The model under review builds one solid part; all positions refer to its coordinate system, in mm. A direction names the side the tool comes from. Round coordinates to 2 decimals unless told otherwise and drop trailing zeros. Order: outer loops, then holes, each group sorted by start corner. A loop starts at its lowest first (then second) coordinate and runs counter-clockwise, first axis right, second up.
1) Clearance check with flat-ended pins moving along their axes: P1, Ø10, axis at x = 55, z = -89.5, coming from the +Y side; P2, Ø0.9, axis at x = -4, y = 0, coming from the +Z side; P3, Ø4.5, axis at y = 14, z = -78.5, coming from the +X side. State where each tip first meets the part, or that it passes through.
2) Consider section A-A (y = 20.75). Give the number of separate pieces and of enclosed holes in the cut face, then the cut area to 3 significant figures.
3) Mouldability with a two-part tool opening along Z and no side actions: class faces 1 (the face through (0, -1, -83)), 2 (the face through (-25.27, 12.08, -93.65)), 3 (the face through (24.94, 12.08, -93.74)), 4 (the face through (-1, -3, -87)) as pulls with the +Z half, pulls with the -Z half, needs draft (parallel to the pull), parting line crosses it, or undercut.
4) Consider section B-B (x = 8). Give the boundary of the cut face in (y, z), then the cut area to 3 significant figures.
5) To check wall thickness, follow L1, parallel to X at y = 4, z = -74; L2, parallel to X at y = 11.5, z = -69.5; L3, parallel to X at y = 1.5, z = -84. State the ranges of each line that lie inside material, in increasing order.
6) Machinability: for faces 5 (the face through (-25.7, 10.56, -96.64)), 6 (the face through (-36.139, 12.078, -88.594)), 7 (the face through (33, 12, -71)), 8 (the face through (-62.19, 10.94, -81.72)), 9 (the face through (-19, 11, -74)), which of the approach directions +Z, -Z, +X, -X, +Y, -Y give a long, thin tool a straight path to every point of the face, cutting with its end or side? Answer none if there is none.
from build123d import *

# Parameters (mm, degrees)
EXTRUDE_1842_DEPTH     = 3
SKETCH_5_W             = 14
SKETCH_5_H             = 12
EXTRUDE_4250_DEPTH     = 24.5
SKETCH_9_W             = 22
SKETCH_9_H             = 11
EXTRUDE_5165_DEPTH     = 2
SKETCH_11_W            = 22
SKETCH_11_H            = 7
CUT_EXTRUDE_6076_DEPTH = 3
SKETCH_6_R             = 2
CUT_EXTRUDE_6516_DEPTH = 127.101149876
FILLET_2_R             = 6


with BuildPart() as part:
    # 草图1 → Extrude 1842 (new body)
    with BuildSketch(Plane(origin=(0, 0, 0), x_dir=(1, 0, 0), z_dir=(0, 1, 0))):
        with BuildLine():
            Line((-65, 75.993420768), (-65, 68))
            Line((-65, 68), (-19, 68))
            Line((-19, 68), (-19, 83))
            Line((-19, 83), (19, 83))
            Line((19, 83), (19, 68))
            Line((19, 68), (65, 68))
            Line((65, 68), (65, 75.993420768))
            ThreePointArc((65, 75.993420768), (62.939630568, 77.708448086), (60.834029942, 79.367630688))
            Line((60.834029942, 79.367630688), (63.508330249, 83.999654695))
            Line((63.508330249, 83.999654695), (40.991669751, 96.999654695))
            Line((40.991669751, 96.999654695), (38.317369443, 92.367630688))
            ThreePointArc((38.317369443, 92.367630688), (25.88190451, 96.592582629), (13, 99.151399385))
            Line((13, 99.151399385), (13, 104.5))
            Line((13, 104.5), (-13, 104.5))
            Line((-13, 104.5), (-13, 99.151399385))
            ThreePointArc((-13, 99.151399385), (-25.88190451, 96.592582629), (-38.317369443, 92.367630688))
            Line((-38.317369443, 92.367630688), (-40.991669751, 96.999654695))
            Line((-40.991669751, 96.999654695), (-63.508330249, 83.999654695))
            Line((-63.508330249, 83.999654695), (-60.834029942, 79.367630688))
            ThreePointArc((-60.834029942, 79.367630688), (-62.939630568, 77.708448086), (-65, 75.993420768))
        make_face()
    extrude(amount=-EXTRUDE_1842_DEPTH)

    # 草图5 → Extrude 4250 (add)
    with BuildSketch(Plane(origin=(0, 0, 0), x_dir=(1, 0, 0), z_dir=(0, 1, 0))):
        with BuildLine():
            Line((-11, 104.5), (-13, 104.5))
            Line((-13, 104.5), (-13, 99.151399385))
            ThreePointArc((-13, 99.151399385), (-25.88190451, 96.592582629), (-38.317369443, 92.367630688))
            Line((-38.317369443, 92.367630688), (-40.991669751, 96.999654695))
            Line((-40.991669751, 96.999654695), (-42.723720558, 95.999654695))
            Line((-42.723720558, 95.999654695), (-37.223720558, 86.473375254))
            Line((-37.223720558, 86.473375254), (-35.491669751, 87.473375254))
            Line((-35.491669751, 87.473375254), (-36.804129114, 89.746621553))
            ThreePointArc((-36.804129114, 89.746621553), (-25.105447375, 93.69480515), (-13, 96.124918726))
            Line((-13, 96.124918726), (-13, 93.5))
            Line((-13, 93.5), (-11, 93.5))
            Line((-11, 93.5), (-11, 104.5))
        make_face()
        with BuildLine():
            Line((13, 104.5), (11, 104.5))
            Line((11, 104.5), (11, 93.5))
            Line((11, 93.5), (13, 93.5))
            Line((13, 93.5), (13, 96.124918726))
            ThreePointArc((13, 96.124918726), (25.105447375, 93.69480515), (36.804129114, 89.746621553))
            Line((36.804129114, 89.746621553), (35.491669751, 87.473375254))
            Line((35.491669751, 87.473375254), (37.223720558, 86.473375254))
            Line((37.223720558, 86.473375254), (42.723720558, 95.999654695))
            Line((42.723720558, 95.999654695), (40.991669751, 96.999654695))
            Line((40.991669751, 96.999654695), (38.317369443, 92.367630688))
            ThreePointArc((38.317369443, 92.367630688), (25.88190451, 96.592582629), (13, 99.151399385))
            Line((13, 99.151399385), (13, 104.5))
        make_face()
        with BuildLine():
            Line((-61.776279442, 84.999654695), (-63.508330249, 83.999654695))
            Line((-63.508330249, 83.999654695), (-60.834029942, 79.367630688))
            ThreePointArc((-60.834029942, 79.367630688), (-62.939630568, 77.708448086), (-65, 75.993420768))
            Line((-65, 75.993420768), (-65, 68))
            Line((-65, 68), (-62, 68))
            Line((-62, 68), (-62, 74.598927606))
            ThreePointArc((-62, 74.598927606), (-60.669899006, 75.684630901), (-59.320789612, 76.746621553))
            Line((-59.320789612, 76.746621553), (-58.008330249, 74.473375254))
            Line((-58.008330249, 74.473375254), (-56.276279442, 75.473375254))
            Line((-56.276279442, 75.473375254), (-61.776279442, 84.999654695))
        make_face()
        with BuildLine():
            Line((58.008330249, 74.473375254), (59.320789612, 76.746621553))
            ThreePointArc((59.320789612, 76.746621553), (60.669899006, 75.684630901), (62, 74.598927606))
            Line((62, 74.598927606), (62, 68))
            Line((62, 68), (65, 68))
            Line((65, 68), (65, 75.993420768))
            ThreePointArc((65, 75.993420768), (62.939630568, 77.708448086), (60.834029942, 79.367630688))
            Line((60.834029942, 79.367630688), (63.508330249, 83.999654695))
            Line((63.508330249, 83.999654695), (61.776279442, 84.999654695))
            Line((61.776279442, 84.999654695), (56.276279442, 75.473375254))
            Line((56.276279442, 75.473375254), (58.008330249, 74.473375254))
        make_face()
        with Locations((-26, 74)):
            Rectangle(SKETCH_5_W, SKETCH_5_H)
        with Locations((26, 74)):
            Rectangle(SKETCH_5_W, SKETCH_5_H)
    extrude(amount=EXTRUDE_4250_DEPTH)

    # 草图9 → Extrude 5165 (add)
    with BuildSketch(Plane(origin=(0, 0, 0), x_dir=(1, 0, 0), z_dir=(0, 1, 0))):
        Polygon((-56.276279442, 75.473375254), (-37.223720558, 86.473375254), (-42.723720558, 95.999654695), (-61.776279442, 84.999654695), align=None)
        with Locations((0, 99)):
            Rectangle(SKETCH_9_W, SKETCH_9_H)
        Polygon((37.223720558, 86.473375254), (56.276279442, 75.473375254), (61.776279442, 84.999654695), (42.723720558, 95.999654695), align=None)
    extrude(amount=EXTRUDE_5165_DEPTH)

    # 草图11 → Cut-Extrude 6076 (cut)
    with BuildSketch(Plane(origin=(0, 2, 0), x_dir=(1, 0, 0), z_dir=(0, 1, 0))):
        Polygon((-60.776279442, 83.267603888), (-41.723720558, 94.267603888), (-38.223720558, 88.205426061), (-57.276279442, 77.205426061), align=None)
        with Locations((0, 99)):
            Rectangle(SKETCH_11_W, SKETCH_11_H)
        Polygon((41.723720558, 94.267603888), (60.776279442, 83.267603888), (57.276279442, 77.205426061), (38.223720558, 88.205426061), align=None)
    extrude(amount=-CUT_EXTRUDE_6076_DEPTH, mode=Mode.SUBTRACT)

    # 草图6 → Cut-Extrude 6516 (cut, through all)
    with BuildSketch(Plane.XZ.offset(3)):
        with Locations(Location((-26, -74, 0), (0, 0, 270))):
            Circle(SKETCH_6_R)
        with Locations(Location((26, -74, 0), (0, 0, 270))):
            Circle(SKETCH_6_R)
    extrude(amount=-CUT_EXTRUDE_6516_DEPTH, mode=Mode.SUBTRACT)

    # 圆角2
    fillet_2_edges = [part.edges().sort_by_distance(p)[0] for p in [
        (-33, 12.25, -80),
        (33, 12.25, -80),
    ]]
    fillet(fillet_2_edges, radius=FILLET_2_R)


solid = part.part
Answer below:
1. P1: stops at y = 2
1. P2: stops at z = -83
1. P3: stops at x = 64.7
2. separate pieces: 6
2. enclosed holes: 2
2. area: 651 mm2
3. face 1: pulls with the +Z half
3. face 2: undercut
3. face 3: undercut
3. face 4: needs draft
4. outline: (-3, -104.5) - (2, -104.5) - (2, -102.5) - (-1, -102.5) - (-1, -95.5) - (2, -95.5) - (2, -93.5) - (0, -93.5) - (0, -83) - (-3, -83) - close
4. area: 65.5 mm2
5. L1: x = -65 to -62, -33 to -28, -24 to -19, 19 to 24, 28 to 33, 62 to 65
5. L2: x = -65 to -62, -33 to -19, 19 to 33, 62 to 65
5. L3: x = -63.51 to -59.51, -45.51 to -41.51, 41.51 to 45.51, 59.51 to 63.51
6. face 5: -Z, +Y, -Y
6. face 6: +Y
6. face 7: +Z, +Y
6. face 8: -X, +Y, -Y
6. face 9: +Z, +Y, -Y
